```python
from build123d import *

# Parameters (mm, degrees)
SKETCH_1_W          = 30
SKETCH_1_H          = 30
EXTRUDE_1_DEPTH     = 7
SKETCH_5_R          = 13.083
SKETCH_5_R_2        = 11.083
CUT_EXTRUDE_1_DEPTH = 5.8


with BuildPart() as part:
    # 草图1 → 凸台-拉伸1 (new body)
    with BuildSketch(Plane.XY):
        with Locations((15, -15)):
            Rectangle(SKETCH_1_W, SKETCH_1_H)
    extrude(amount=EXTRUDE_1_DEPTH)

    # 草图5 → 切除-拉伸1 (cut)
    with BuildSketch(Plane.XY.offset(7)):
        with Locations((15, -15.083)):
            Circle(SKETCH_5_R)
        with Locations((15, -15.083)):
            Circle(SKETCH_5_R_2, mode=Mode.SUBTRACT)
    extrude(amount=-CUT_EXTRUDE_1_DEPTH, mode=Mode.SUBTRACT)


solid = part.part
```
The model under review builds one solid part; all positions refer to its coordinate system, in mm. A direction names the side the tool comes from. Round coordinates to 2 decimals unless told otherwise and drop trailing zeros. Loops run counter-clockwise (first coordinate to the right, second up) from the corner with the lowest first, then second, coordinate; pieces in that order, holes last. Notation, with made-up numbers: (45.25, -24) -> (70.25, -24) arc R35 cw to (70.25, 13) -> close; hole circle Ø10 at (78, 66). An arc over 180 degrees is marked (long way). Answer as a JSON object with one key per item and string values. Group by question number.
1) We need section A-A on x = 15. Write out the cut boundary in (y, z).
2) We need section B-B on z = 2.5. Write out the cut boundary in (x, y), then the cut area to 3 significant figures.
3) For line 1 (Y direction, x = 15, z = 3.8); line 2 (Y direction, x = 13.75, z = 2); line 3 (X direction, y = -14.25, z = 4), list the stretches that pass through material, from the lowest coordinate up. Write a range as [from, to].
4) For faces 1 (the face through (30, -15, 3)), 2 (the face through (27.479, -11.153, 4.141)), list the 3-axis set-ups (+Z, -Z, +X, -X, +Y, -Y) from which the entire face can be reached by the end or side of a thin tool; tool diameter is ignored.
5) We need section C-C on y = -18.75. Write out the cut boundary in (x, z), then the cut area to 3 significant figures.
Result set:
{
 "1": {"outline": "(-30, 0) -> (0, 0) -> (0, 7) -> (-2, 7) -> (-2, 1.2) -> (-4, 1.2) -> (-4, 7) -> (-26.17, 7) -> (-26.17, 1.2) -> (-28.17, 1.2) -> (-28.17, 7) -> (-30, 7) -> close"},
 "2": {"outline": "(0, -30) -> (30, -30) -> (30, 0) -> (0, 0) -> close; circle Ø22.17 at (15, -15.08); hole circle Ø26.17 at (15, -15.08)", "area": "748 mm²"},
 "3": {"line 1": "[-30, -28.17], [-26.17, -4], [-2, 0]", "line 2": "[-30, -28.11], [-26.1, -4.07], [-2.06, 0]", "line 3": "[0, 1.94], [3.95, 26.05], [28.06, 30]"},
 "4": {"face 1": "+Z, -Z, +X, +Y, -Y", "face 2": "+Z"},
 "5": {"outline": "(0, 0) -> (30, 0) -> (30, 7) -> (27.56, 7) -> (27.56, 1.2) -> (25.46, 1.2) -> (25.46, 7) -> (4.54, 7) -> (4.54, 1.2) -> (2.44, 1.2) -> (2.44, 7) -> (0, 7) -> close", "area": "186 mm²"}
}
